Could you check a few things on this model? Use its own coordinates, in mm. A direction names the side the tool comes from. Round coordinates to 2 decimals unless told otherwise and drop trailing zeros. Loops run counter-clockwise (first coordinate to the right, second up) from the corner with the lowest first, then second, coordinate; pieces in that order, holes last. Notation, with made-up numbers: (-3.75, 38.5) -> (1.25, 38.5) arc R4 ccw to (1.25, 44.5) -> close; hole circle Ø4 at (40, 79.5). An arc over 180 degrees is marked (long way). Put each result on its own line as item: value. Start each with the question number.
1. Imagine slicing it at D-D, the plane y = -2.5. Please give me the cut outline in (x, z).
2. Imagine slicing it at B-B, the plane z = 22. Please give me the cut outline in (x, y).
3. Which directions (+Z, -Z, +X, -X, +Y, -Y) give clear straight access to the entire face, cutting with the end or side of a thin tool? Please do faces 1 (the flat face through (-13, 0, 18)), 2 (the flat face through (-19, 6, 0)), 3 (the flat face through (8.6, 25.1, 31.242)), 4 (the flat face through (-23, -17.297, 7)), 5 (the flat face through (-22, 28.767, 7)).
4. If we mould it in two halves opening along Y, with no side actions, what happens to faces 6 (the flat face through (-13, 11.938, 19)), 7 (the flat face through (-52.353, 6, 7)), 8 (the cylindrical face through (30.72, 11.56, 15.84))? For each: pulls with the +Y half, pulls with the -Y half, needs draft (parallel to the pull), parting line crosses it, or undercut.
5. I need wall thicknesses on line 1 (X direction, y = 18.5, z = 12); line 2 (X direction, y = -4, z = 6); line 3 (Z direction, x = -17.5, y = 18.5). Which ranges of each line are inside material? Lowest first, please. Write a range as [from, to].
6. Imagine slicing it at C-C, the plane x = 4. Please give me the cut outline in (y, z), and give its area (3 significant figures).
7. Imagine slicing it at A-A, the plane y = 8.5. Please give me the cut outline in (x, z), and give its area (3 significant figures).
8. I'm going to push flat-ended pins straight in: P1, Ø1.5, axis at x = -30, z = 10.5, coming from the +Y side; P2, Ø1.5, axis at x = -7, z = 8, coming from the -Y side; P3, Ø9, axis at x = -16.5, z = 19.5, coming from the -Y side; P4, Ø3, axis at x = -24, z = 17, coming from the +Y side. Where does each tip first touch, or does it pass through?
```python
from build123d import *

# Parameters (mm, degrees)
F1_DEPTH = 13.716
F2_DEPTH = 31.242
F3_R     = 19.40346
F4_DEPTH = 44.45
F6_DEPTH = 11.938


with BuildPart() as f1:
    # F0 (on Top) → F1 (new body)
    with BuildSketch(Plane.XY):
        with BuildLine():
            Line((6.759355, 28.766602), (-52.353363, 28.766602))
            Line((-52.353363, 28.766602), (-52.353363, -17.296961))
            Line((-52.353363, -17.296961), (6.759355, -17.296961))
            ThreePointArc((6.759355, -17.296961), (-11.458258, 5.734821), (6.759355, 28.766602))
        make_face()
    extrude(amount=F1_DEPTH)

    # F0 (on Top) → F2 (join)
    with BuildSketch(Plane.XY):
        with BuildLine():
            ThreePointArc((35.877493, 5.734821), (26.892468, 24.297747), (6.759355, 28.766602))
            Line((6.759355, 28.766602), (12.209618, 28.766602))
            Line((12.209618, 28.766602), (12.209618, -17.296961))
            Line((12.209618, -17.296961), (6.759355, -17.296961))
            ThreePointArc((6.759355, -17.296961), (26.892468, -12.828105), (35.877493, 5.734821))
        make_face()
        with BuildLine():
            Line((12.209618, 28.766602), (6.759355, 28.766602))
            ThreePointArc((6.759355, 28.766602), (-11.458258, 5.734821), (6.759355, -17.296961))
            Line((6.759355, -17.296961), (12.209618, -17.296961))
            Line((12.209618, -17.296961), (12.209618, 28.766602))
        make_face()
    extrude(amount=F2_DEPTH)

    # F3 (on face) → F4 (cut)
    with BuildSketch(Plane.XY.offset(31.242)):
        with Locations((12.209618, 5.734821)):
            Circle(F3_R)
    extrude(amount=-F4_DEPTH, mode=Mode.SUBTRACT)

    # F5 (on Front) → F6 (join)
    with BuildSketch(Plane.XZ):
        Polygon((-10.565767, 13.289291), (-10.565767, 30.780276), (-18.974263, 13.289291), align=None)
    extrude(amount=-F6_DEPTH)


solid = f1.part
```
Entries:
1. outline: (-52.35, 0) -> (-5.36, 0) -> (-5.36, 31.24) -> (-9.98, 31.24) -> (-9.98, 13.72) -> (-52.35, 13.72) -> close; (29.78, 0) -> (34.4, 0) -> (34.4, 31.24) -> (29.78, 31.24) -> close
2. outline: (-14.79, 0) -> (-10.75, 0) arc R23.67 ccw to (6.76, -17.3) arc R23.67 ccw to (35.88, 5.73) arc R23.67 ccw to (-10.63, 11.94) -> (-14.79, 11.94) -> close; hole circle Ø38.81 at (12.21, 5.73)
3. face 1: +Z, -X, -Y
3. face 2: -Z, +X, -X, +Y, -Y
3. face 3: +Z, +X, -X, +Y, -Y
3. face 4: +Z, -Z, -X, -Y
3. face 5: +Z, -Z, -X, +Y
4. face 6: pulls with the +Y half
4. face 7: needs draft
4. face 8: undercut
5. line 1: [-52.35, -2.4], [26.82, 32.14]
5. line 2: [-52.35, -4.58], [28.99, 33.78]
5. line 3: [0, 13.72]
6. outline: (-17.3, 0) -> (-11.85, 0) -> (-11.85, 31.24) -> (-16.46, 31.24) -> (-16.46, 13.72) -> (-17.3, 13.72) -> close; (23.32, 0) -> (28.77, 0) -> (28.77, 13.72) -> (27.93, 13.72) -> (27.93, 31.24) -> (23.32, 31.24) -> close
6. area: 311 mm^2
7. outline: (-52.35, 0) -> (-7, 0) -> (-7, 31.24) -> (-11.3, 31.24) -> (-11.3, 29.26) -> (-18.77, 13.72) -> (-52.35, 13.72) -> close; (31.42, 0) -> (35.72, 0) -> (35.72, 31.24) -> (31.42, 31.24) -> close
7. area: 890 mm^2
8. P1: y = 28.77
8. P2: y = -17.3
8. P3: y = 0
8. P4: through
